Autodesk Inventor part; units mm, degrees
ref_plane "YZ Plane" through (0, 0, 0) normal (1, 0, 0) x (0, 1, 0)
ref_plane "XZ Plane" through (0, 0, 0) normal (0, 1, 0) x (-1, 0, 0)
ref_plane "XY Plane" through (0, 0, 0) normal (0, 0, 1) x (1, 0, 0)
sketch "Sketch1" plane through (0, 0, 0) normal (0, 1, 0) x (-1, 0, 0)
  line L0 (-10.75, 10.5) -> (10.75, 10.5)
  line L1 (10.75, 10.5) -> (10.75, -10.5)
  line L2 (10.75, -10.5) -> (-10.75, -10.5)
  line L3 (-10.75, -10.5) -> (-10.75, 10.5)
  line L4 (-10.75, 10.5) -> (10.75, -10.5) construction
  line L5 (10.75, 10.5) -> (-10.75, -10.5) construction
  circle A0 centre (0, 0) radius 6.1
  line L6 (0, 0) -> (9, 0) construction
  line L7 (0, 0) -> (9, 0) construction
  line L8 (0, 0) -> (10.2, 0) construction
  line L9 (0, 0) -> (9, 0) construction
  line L10 (0, 0) -> (10.2, 0)
  line L11 (0, 0) -> (5.1, 8.8335) construction
  line L12 (0, 0) -> (-5.1, 8.8335) construction
  line L13 (0, 0) -> (-10.2, 0) construction
  line L14 (0, 0) -> (-5.1, -8.8335) construction
  line L15 (0, 0) -> (5.1, -8.8335) construction
  line L16 (10.35, -0.2598) -> (5.4, -8.8335)
  line L17 (5.4, -8.8335) -> (-5.1, -8.8335)
  line L18 (-5.1, -8.8335) -> (-10.2, 0)
  line L19 (-10.2, 0) -> (-5.1, 8.8335)
  line L20 (-5.1, 8.8335) -> (5.1, 8.8335)
  line L21 (5.1, 8.8335) -> (10.35, -0.2598)
  dimension "d0" = 21.5
  dimension "d1" = 21
  dimension "d2" = 12.2
  dimension "d28" = 10.2
  dimension "d31" = 360
extrude "Extrusion1" add sketch "Sketch1" along normal blind 3 contours L0 L1 L2 L3 | A0 | L21 L16 L17 L18 L19 L20
extrude "Extrusion6" cut sketch "Sketch1" along normal blind 12.2 contours A0 | L21 L16 L17 L18 L19 L20
extrude "Extrusion7" add sketch "Sketch1" along normal blind 1 contours L21 L16 L17 L18 L19 L20
equation "\"d33\" = d2"
properties part number "ScrewTest"
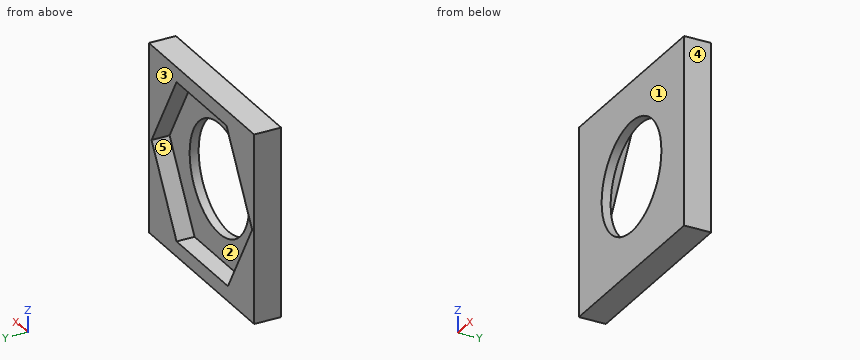
Could you check a few things on this model? Use its own coordinates, in mm. Face numbers are marked on the shaded views. A direction names the side the tool comes from. Give positions to 0.01 mm unless a question says otherwise; leave off trailing zeros. Loops run counter-clockwise (first coordinate to the right, second up) from the corner with the lowest first, then second, coordinate; pieces in that order, holes last. Notation, with made-up numbers: (28, 46) -> (41, 46) arc R18 cw to (41, 58) -> close; hole circle Ø4 at (51, 18). An arc over 180 degrees is marked (long way). Return JSON: item names as keys, results as strings.
Item 1: I need wall thicknesses on L1, parallel to Z at x = 0, y = 0.65; L2, parallel to Z at x = 3.25, y = 2.25; L3, parallel to Y at x = -2.5, z = 6. Which ranges of each line are inside material? Lowest first, please. Write a range as from..to.
Geometry results:
{"L1": "z = -10.5..-6.1, 6.1..10.5", "L2": "z = -10.5..-8.83, 8.83..10.5", "L3": "y = 0..1"}
Item 2: If we section it at D-D on x = -7.75: List the corners of the cut face in (y, z) for me, plus the area to 3 significant figures.
Geometry results:
{"outline": "(0, -10.5) -> (3, -10.5) -> (3, -4.76) -> (1, -4.76) -> (1, 4.24) -> (3, 4.24) -> (3, 10.5) -> (0, 10.5) -> close", "area": "45.0 mm²"}
Item 3: If we section it at B-B on y = 0.4: List the corners of the cut face in (x, z) for me.
Geometry results:
{"outline": "(-10.75, -10.5) -> (10.75, -10.5) -> (10.75, 10.5) -> (-10.75, 10.5) -> close; hole circle Ø12.2 at (0, 0)"}
Item 4: If we section it at C-C on z = 4.5: List the corners of the cut face in (x, y) for me.
Geometry results:
{"outline": "(-10.75, 0) -> (-4.12, 0) -> (-4.12, 1) -> (-7.6, 1) -> (-7.6, 3) -> (-10.75, 3) -> close; (4.12, 0) -> (10.75, 0) -> (10.75, 3) -> (7.6, 3) -> (7.6, 1) -> (4.12, 1) -> close"}
Item 5: We'd pull the mould along X, two halves only. Please class the marked faces 3, 4 and 5: +X half, -X half, draft (parallel to the pull), parting line (faces both ways), or undercut.
Geometry results:
{"face 3": "draft", "face 4": "+X half", "face 5": "undercut"}
Item 6: I'm going to push flat-ended pins straight in: pin 1 (5.5 mm diameter, centred on x = -1, z = -4, fed in from +Y); pin 2 (10 mm diameter, centred on x = 2, z = 6.5, fed in from +Y). Where does each tip first touch, or does it pass through?
Geometry results:
{"pin 1": "stops at y = 1", "pin 2": "stops at y = 3"}
Item 7: Which directions (+Z, -Z, +X, -X, +Y, -Y) give clear straight access to the entire face, cutting with the end or side of a thin tool? Please do the marked faces 1 and 2.
Geometry results:
{"face 1": "+Z, -Z, +X, -X, -Y", "face 2": "+Y"}
Item 8: If we section it at A-A on x = 0: List the corners of the cut face in (y, z) for me.
Geometry results:
{"outline": "(0, -10.5) -> (3, -10.5) -> (3, -8.83) -> (1, -8.83) -> (1, -6.1) -> (0, -6.1) -> close; (0, 6.1) -> (1, 6.1) -> (1, 8.83) -> (3, 8.83) -> (3, 10.5) -> (0, 10.5) -> close"}
